For this review, take the finished solid that the model builds, in its own axes (mm). Face numbers are marked on the shaded views. A direction names the side the tool comes from. Round coordinates to 2 decimals unless told otherwise and drop trailing zeros. Loops run counter-clockwise (first coordinate to the right, second up) from the corner with the lowest first, then second, coordinate; pieces in that order, holes last.
1. Tool access review of the marked faces 4, 5 and 6: name each direction out of +Z, -Z, +X, -X, +Y, -Y from which nothing blocks a thin tool from reaching the whole face with its end or side.
2. Clearance check with flat-ended pins moving along their axes: pin 1 Ø4 at (y, z) = (19.5, -12.5) entering from -X; pin 2 Ø6 at (x, y) = (-5.5, 24) entering from +Z; pin 3 Ø13 at (x, z) = (-47, 46.5) entering from +Y; pin 4 Ø25 at (x, z) = (9.5, 0) entering from +Y. State where each tip first meets the part, or that it passes through.
3. Consider section D-D on z = -29. State the section outline as (x, y) points, then the cut area to 3 significant figures.
4. To check wall thickness, follow line 1 along Z through (x, y) = (0, 3.5); line 2 along Y through (x, z) = (67.5, -8.5); line 3 along Z through (x, y) = (46.5, 34.5). State the ranges of each line that lie inside material, in increasing order.
5. Draft analysis for pull direction X (two halves, no side actions). For the marked faces 1, 2 and 3, state which applies: released by +X, released by -X, zero draft, split by the parting line, or undercut.
6. Consider section C-C on x = 0. State the section outline as (y, z) points, then the cut area to 3 significant figures.
7. Consider section B-B on y = 4.5. State the section outline as (x, z) points.
8. Consider section A-A on z = 0. State the section outline as (x, y) points, then the cut area to 3 significant figures.
from build123d import *

# Parameters (mm, degrees)
HOLE1_D                 = 50
HOLE1_CBORE_D           = 84
HOLE1_CBORE_DEPTH       = 9
HOLE2_D                 = 84
HOLE2_DEPTH             = 24.5
BOSS_EXTRUDE1_DEPTH     = 24
CIRPATTERN1_COUNT       = 4
HOLE3_D                 = 12
HOLE3_DEPTH             = 24.5
CUT_EXTRUDE2_DEPTH      = 24
CIRPATTERN2_COUNT       = 2
CUT_EXTRUDE3_DEPTH      = 147.482080815
CUT_EXTRUDE3_DEPTH_BACK = 147.482080815
SKETCH12_W              = 6
SKETCH12_H              = 6


with BuildPart() as part:
    # Sketch1 → Revolve1 (revolve)
    with BuildSketch(Plane.XY, mode=Mode.PRIVATE) as revolve1_sk:
        Polygon((0, 0), (0, 39), (-52, 39), (-52, 11), (-100, 11), (-100, 0), align=None)
    revolve(revolve1_sk.sketch.rotate(Axis((0, 0, 0), (0, 1, 0)), 270), axis=Axis((0, 0, 0), (0, 1, 0)))

    # Hole1 (through all)
    with Locations(Plane(origin=(0, 39, 0), x_dir=(1, 0, 0), z_dir=(0, 1, 0))):
        with Locations((0, 0)):
            CounterBoreHole(HOLE1_D / 2, HOLE1_CBORE_D / 2, HOLE1_CBORE_DEPTH)

    # Hole2
    with Locations(Plane(origin=(0, 0, 0), x_dir=(-1, 0, 0), z_dir=(0, -1, 0))):
        with Locations((0, 0)):
            Hole(HOLE2_D / 2, depth=HOLE2_DEPTH)

    # Sketch8 → Boss-Extrude1 (add)
    with BuildSketch(Plane(origin=(0, 11, 0), x_dir=(1, 0, 0), z_dir=(0, 1, 0))):
        with BuildLine():
            Line((25.512367483, 45.311357356), (36.062445841, 55.861435714))
            ThreePointArc((36.062445841, 55.861435714), (55.861435714, 55.861435714), (55.861435714, 36.062445841))
            Line((55.861435714, 36.062445841), (45.311357356, 25.512367483))
            ThreePointArc((45.311357356, 25.512367483), (36.769552622, 36.769552622), (25.512367483, 45.311357356))
        make_face()
    boss_extrude1 = extrude(amount=BOSS_EXTRUDE1_DEPTH)

    # CirPattern1: Boss-Extrude1 ×4 about axis
    cirpattern1_axis = Axis((0, 0, 0), (0, 1, 0))
    for i in range(1, CIRPATTERN1_COUNT):
        add(boss_extrude1.rotate(cirpattern1_axis, i * 360 / CIRPATTERN1_COUNT))

    # Hole3
    with Locations(Plane(origin=(0, 35, 0), x_dir=(1, 0, 0), z_dir=(0, 1, 0))):
        with Locations((45.961940777, 45.961940777), (45.961940777, -45.961940777), (-45.961940777, -45.961940777), (-45.961940777, 45.961940777)):
            Hole(HOLE3_D / 2, depth=HOLE3_DEPTH)

    # Sketch11 → Cut-Extrude2 (cut)
    with BuildSketch(Plane(origin=(0, 11, 0), x_dir=(1, 0, 0), z_dir=(0, 1, 0))):
        with BuildLine():
            Line((80, 8), (120, 8))
            ThreePointArc((120, 8), (128, 0), (120, -8))
            Line((120, -8), (80, -8))
            ThreePointArc((80, -8), (72, 0), (80, 8))
        make_face()
    cut_extrude2 = extrude(amount=-CUT_EXTRUDE2_DEPTH, mode=Mode.SUBTRACT)

    # CirPattern2: Cut-Extrude2 ×2 about axis
    cirpattern2_axis = Axis((0, 0, 0), (0, 1, 0))
    for i in range(1, CIRPATTERN2_COUNT):
        add(cut_extrude2.rotate(cirpattern2_axis, i * 360 / CIRPATTERN2_COUNT), mode=Mode.SUBTRACT)

    # Sketch12 → Cut-Extrude3 (cut, two sides: drawn at the far end of the back side and taken through both)
    with BuildSketch(Plane(origin=(0, 0, 0), x_dir=(0, 0, -1), z_dir=(1, 0, 0)).offset(-CUT_EXTRUDE3_DEPTH_BACK)):
        with Locations((-10, 14)):
            Rectangle(SKETCH12_W, SKETCH12_H)
        with Locations((10, 14)):
            Rectangle(SKETCH12_W, SKETCH12_H)
    extrude(amount=CUT_EXTRUDE3_DEPTH + CUT_EXTRUDE3_DEPTH_BACK, mode=Mode.SUBTRACT)


solid = part.part
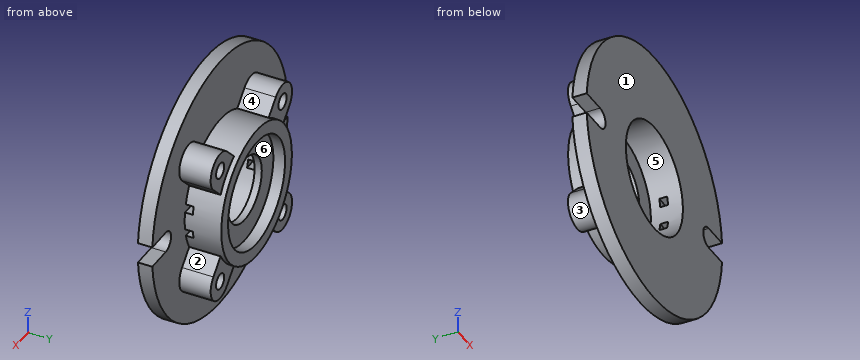
Resolved:
1. face 4: +Z, +Y
1. face 5: -Y
1. face 6: +Y
2. pin 1: stops at x = -50.93
2. pin 2: stops at z = 51.94
2. pin 3: stops at y = 35
2. pin 4: passes through
3. outline: (-95.7, 0) - (-30.38, 0) - (-30.38, 24.5) - (30.38, 24.5) - (30.38, 0) - (95.7, 0) - (95.7, 11) - (48.8, 11) - (48.8, 35) - (43.16, 35) - (43.16, 39) - (30.38, 39) - (30.38, 30) - (-30.38, 30) - (-30.38, 39) - (-43.16, 39) - (-43.16, 35) - (-48.8, 35) - (-48.8, 11) - (-95.7, 11) - close
3. area: 2,760 mm2
4. line 1: z = -100 to -42, 42 to 100
4. line 2: y = 0 to 11
4. line 3: z = -59.95 to -51.94, -39.99 to -26.7, -23.28 to 23.28, 26.7 to 39.99, 51.94 to 59.95
5. face 1: zero draft
5. face 2: released by +X
5. face 3: undercut
6. outline: (0, -100) - (11, -100) - (11, -52) - (39, -52) - (39, -42) - (30, -42) - (30, -25) - (24.5, -25) - (24.5, -42) - (0, -42) - close; (0, 42) - (24.5, 42) - (24.5, 25) - (30, 25) - (30, 42) - (39, 42) - (39, 52) - (11, 52) - (11, 100) - (0, 100) - close
6. area: 2,020 mm2
7. outline: (-99.68, -8) arc R100 ccw to (99.68, -8) - (80, -8) arc R8 cw to (80, 8) - (99.68, 8) arc R100 ccw to (-99.68, 8) - (-80, 8) arc R8 cw to (-80, -8) - close; hole circle Ø84 at (0, 0)
8. outline: (-72, 0) - (-42, 0) - (-42, 24.5) - (-25, 24.5) - (-25, 30) - (-42, 30) - (-42, 39) - (-52, 39) - (-52, 11) - (-72, 11) - close; (25, 24.5) - (42, 24.5) - (42, 0) - (72, 0) - (72, 11) - (52, 11) - (52, 39) - (42, 39) - (42, 30) - (25, 30) - close
8. area: 1,410 mm2
